The listing builds one solid part. Answer for the finished solid, in the listing's coordinates (mm). Coordinates: 2 decimals unless noted, no trailing zeros. Order: outer loops, then holes, each group sorted by start corner. A loop starts at its lowest first (then second) coordinate and runs counter-clockwise, first axis right, second up. Notation, with made-up numbers: (42.5, -9) -> (73.5, -9) arc R30 ccw to (73.5, 18) -> close; hole circle Ø6 at (0.25, 59). An arc over 180 degrees is marked (long way). Answer in a Markdown table with one row per item.
```python
from build123d import *

# Parameters (mm, degrees)
SKETCH1_W           = 25.53
SKETCH1_H           = 84
BOSS_EXTRUDE1_DEPTH = 5.15
SKETCH2_W           = 5.106
SKETCH2_H           = 5.15
SKETCH2_W_2         = 5.15
CUT_EXTRUDE1_DEPTH  = 6.15


with BuildPart() as part:
    # Sketch1 → Boss-Extrude1 (new body)
    with BuildSketch(Plane.XY):
        with Locations((12.765, 42)):
            Rectangle(SKETCH1_W, SKETCH1_H)
    extrude(amount=BOSS_EXTRUDE1_DEPTH)

    # Sketch2 → Cut-Extrude1 (cut, through all)
    with BuildSketch(Plane.XY.offset(5.15)):
        with Locations((7.659, 76.275)):
            Rectangle(SKETCH2_W, SKETCH2_H)
        with Locations((17.871, 76.275)):
            Rectangle(SKETCH2_W, SKETCH2_H)
        with Locations((17.878171498, 21.425)):
            Rectangle(SKETCH2_W_2, SKETCH2_H)
        with Locations((7.681, 62.575)):
            Rectangle(SKETCH2_W_2, SKETCH2_H)
        with Locations((17.878171498, 62.575)):
            Rectangle(SKETCH2_W_2, SKETCH2_H)
        with Locations((7.681, 21.425)):
            Rectangle(SKETCH2_W_2, SKETCH2_H)
        with Locations((17.871, 7.725)):
            Rectangle(SKETCH2_W, SKETCH2_H)
        with Locations((7.659, 7.725)):
            Rectangle(SKETCH2_W, SKETCH2_H)
    extrude(amount=-CUT_EXTRUDE1_DEPTH, mode=Mode.SUBTRACT)


solid = part.part
```
(1) Find the intervals of material crossed by line 1 along X through (y, z) = (8.5, 0.7); line 2 along Y through (x, z) = (8, 1.8); line 3 along X through (y, z) = (20, 4.25), in increasing order. Write a range as from..to.
Check values:
| item | result |
|---|---|
| line 1 | 0..5.11, 10.21..15.32, 20.42..25.53 |
| line 2 | 0..5.15, 10.3..18.85, 24..60, 65.15..73.7, 78.85..84 |
| line 3 | 0..5.11, 10.26..15.3, 20.45..25.53 |
(2) A cutting plane is placed at B-B, the plane x = 18. Determine the outline of the cut face in (y, z), then the cut area to 3 significant figures.
Check values:
| item | result |
|---|---|
| outline | (0, 0) -> (5.15, 0) -> (5.15, 5.15) -> (0, 5.15) -> close; (10.3, 0) -> (18.85, 0) -> (18.85, 5.15) -> (10.3, 5.15) -> close; (24, 0) -> (60, 0) -> (60, 5.15) -> (24, 5.15) -> close; (65.15, 0) -> (73.7, 0) -> (73.7, 5.15) -> (65.15, 5.15) -> close; (78.85, 0) -> (84, 0) -> (84, 5.15) -> (78.85, 5.15) -> close |
| area | 327 mm² |
(3) A cutting plane is placed at A-A, the plane y = 21.5. Determine the outline of the cut face in (x, z).
Check values:
| item | result |
|---|---|
| outline | (0, 0) -> (5.11, 0) -> (5.11, 5.15) -> (0, 5.15) -> close; (10.26, 0) -> (15.3, 0) -> (15.3, 5.15) -> (10.26, 5.15) -> close; (20.45, 0) -> (25.53, 0) -> (25.53, 5.15) -> (20.45, 5.15) -> close |
(4) For a pull along X with two mould halves and no side action, classify faces 1 (the flat face through (13, 43, 5.15)), 2 (the flat face through (25.53, 41, 3)), 3 (the flat face through (15.318, 76, 3)), 4 (the flat face through (8, 18.85, 3)) as released by +X, released by -X, zero draft, split by the parting line, or undercut.
Check values:
| item | result |
|---|---|
| face 1 | zero draft |
| face 2 | released by +X |
| face 3 | undercut |
| face 4 | undercut |
(5) A cutting plane is placed at C-C, the plane z = 0.95. Count the separate pieces of the cut face and the enclosed holes in it, then the cut area to 3 significant figures.
Check values:
| item | result |
|---|---|
| separate pieces | 1 |
| enclosed holes | 8 |
| area | 1,930 mm² |
